The drawing under review shows one solid part. Ordinate dimensions are in mm from its lowest x, y, z. Coordinates: 2 decimals unless noted, no trailing zeros. Order: outer loops, then holes, each group sorted by start corner. A loop starts at its lowest first (then second) coordinate and runs counter-clockwise, first axis right, second up. Notation, with made-up numbers: (-18, 58) - (26, 58) arc R13 cw to (26, 69) - close; hole circle Ø2 at (-5, -24.75). An arc over 180 degrees is marked (long way). Answer in a Markdown table with one row per item.
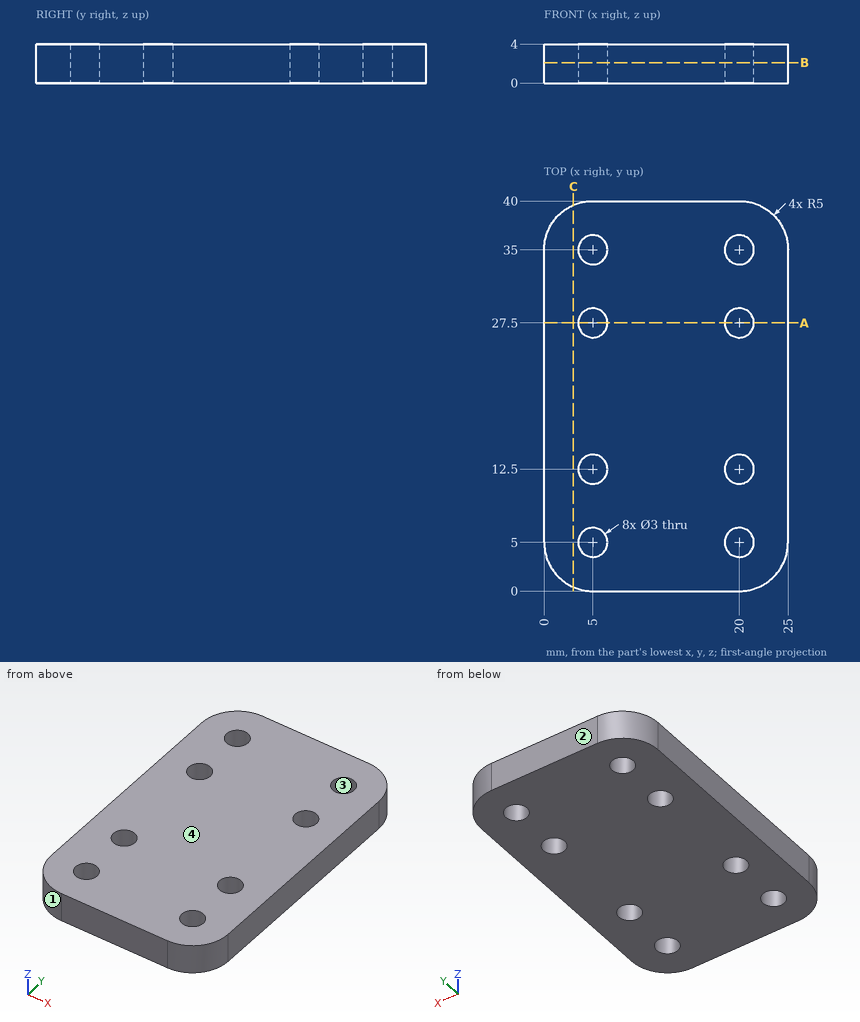
Item 1: We need section A-A, the plane y = 27.5. Write out the cut boundary in (x, z), then the cut area to 3 significant figures.
Check values:
| item | result |
|---|---|
| outline | (0, 0) - (3.5, 0) - (3.5, 4) - (0, 4) - close; (6.5, 0) - (18.5, 0) - (18.5, 4) - (6.5, 4) - close; (21.5, 0) - (25, 0) - (25, 4) - (21.5, 4) - close |
| area | 76.0 mm^2 |
Item 2: We need section B-B, the plane z = 2.1. State how many separate pieces and enclosed holes the cut face has, then the cut area to 3 significant figures.
Check values:
| item | result |
|---|---|
| separate pieces | 1 |
| enclosed holes | 8 |
| area | 922 mm^2 |
Item 3: Clearance check with a flat-ended pin moving along its axis: pin 1 Ø2.5 at (x, y) = (20, 27.5) entering from -Z. State where the tip first meets the part, or that it passes through.
Check values:
| item | result |
|---|---|
| pin 1 | through |
Item 4: Mouldability with a two-part tool opening along Y and no side actions: class the marked faces 1, 2, 3 and 4 as +Y half, -Y half, draft (parallel to the pull), parting line (faces both ways), or undercut.
Check values:
| item | result |
|---|---|
| face 1 | -Y half |
| face 2 | +Y half |
| face 3 | undercut |
| face 4 | draft |
Item 5: To check wall thickness, follow line 1 (Y direction, x = 20, z = 1.35); line 2 (Y direction, x = 6, z = 3.4); line 3 (X direction, y = 38, z = 3.1). State the ranges of each line that lie inside material, in increasing order. Write a range as from..to.
Check values:
| item | result |
|---|---|
| line 1 | 0..3.5, 6.5..11, 14..26, 29..33.5, 36.5..40 |
| line 2 | 0..3.88, 6.12..11.38, 13.62..26.38, 28.62..33.88, 36.12..40 |
| line 3 | 1..24 |
Item 6: We need section C-C, the plane x = 3. Write out the cut boundary in (y, z).
Check values:
| item | result |
|---|---|
| outline | (0.42, 0) - (39.58, 0) - (39.58, 4) - (0.42, 4) - close |
